Can you work these out from the model? Positions are in its coordinate system, mm. A direction names the side the tool comes from. Round coordinates to 2 decimals unless told otherwise and drop trailing zeros. Use a Markdown table: item, result.
from build123d import *

# Parameters (mm, degrees)
EXTRUDE1_DEPTH             = 250
EXTRUDE2_REACH             = 252.071
SKETCH2_R                  = 1.2
SKETCH_R                   = 2.1
SKETCH_R_2                 = 1.2
EXTRUDE4_DEPTH             = 2.3
CHAMFER1_SIZE              = 0.2
LPATTERN1_COUNT            = 17
LPATTERN1_PITCH            = 15
CHAMFER1_OF_LPATTERN1_SIZE = 0.2


with BuildPart() as part:
    # Sketch1 → Extrude1 (new body)
    with BuildSketch(Plane.XY):
        with BuildLine():
            Line((-3.3, -2.4), (3.3, -2.4))
            Line((3.3, -2.4), (3.5, -2.2))
            Line((3.5, -2.2), (3.5, 0.106274607))
            ThreePointArc((3.5, 0.106274607), (3.091294745, 0.282570681), (2.840065792, 0.65))
            Line((2.840065792, 0.65), (2.340065792, 0.65))
            Line((2.340065792, 0.65), (2.340065792, 1.15))
            Line((2.340065792, 1.15), (2.840065792, 1.15))
            ThreePointArc((2.840065792, 1.15), (3.091294745, 1.517429319), (3.5, 1.693725393))
            Line((3.5, 1.693725393), (3.5, 2.2))
            Line((3.5, 2.2), (3.3, 2.4))
            Line((3.3, 2.4), (-3.3, 2.4))
            Line((-3.3, 2.4), (-3.5, 2.2))
            Line((-3.5, 2.2), (-3.5, 1.693725393))
            ThreePointArc((-3.5, 1.693725393), (-3.091294745, 1.517429319), (-2.840065792, 1.15))
            Line((-2.840065792, 1.15), (-2.340065792, 1.15))
            Line((-2.340065792, 1.15), (-2.340065792, 0.65))
            Line((-2.340065792, 0.65), (-2.840065792, 0.65))
            ThreePointArc((-2.840065792, 0.65), (-3.091294745, 0.282570681), (-3.5, 0.106274607))
            Line((-3.5, 0.106274607), (-3.5, -2.2))
            Line((-3.5, -2.2), (-3.3, -2.4))
        make_face()
    extrude(amount=EXTRUDE1_DEPTH)

    # Sketch2 → Extrude2 (cut, up to next)
    with BuildSketch(Plane(origin=(0, 2.4, 0), x_dir=(1, 0, 0), z_dir=(0, 1, 0)), mode=Mode.PRIVATE) as extrude2_sk1:
        with Locations(Location((0, -5, 0), (0, 0, 270))):
            Circle(SKETCH2_R)
    extrude2_tool1 = extrude(extrude2_sk1.sketch, amount=-EXTRUDE2_REACH, mode=Mode.PRIVATE) & part.part
    extrude2 = extrude2_tool1.solids().sort_by_distance((0, 2.4, 5))[0]
    add(extrude2, mode=Mode.SUBTRACT)

    # Sketch → Extrude4 (cut)
    with BuildSketch(Plane(origin=(0, 2.4, 0), x_dir=(1, 0, 0), z_dir=(0, 1, 0))):
        with Locations(Location((0, -5, 0), (0, 0, 270))):
            Circle(SKETCH_R)
        with Locations(Location((0, -5, 0), (0, 0, 270))):
            Circle(SKETCH_R_2, mode=Mode.SUBTRACT)
    extrude4 = extrude(amount=-EXTRUDE4_DEPTH, mode=Mode.SUBTRACT)

    # Chamfer1
    chamfer1_edges = [part.edges().sort_by_distance(p)[0] for p in [
        (0, -2.4, 3.8),
        (0, 2.4, 2.9),
    ]]
    chamfer(chamfer1_edges, length=CHAMFER1_SIZE)

    # LPattern1: Extrude2, Extrude4 ×17
    with Locations(*[(0, 0, i * LPATTERN1_PITCH) for i in range(1, LPATTERN1_COUNT)]):
        add(extrude2, mode=Mode.SUBTRACT)
        add(extrude4, mode=Mode.SUBTRACT)

    # Chamfer1 of LPattern1
    chamfer1_of_lpattern1_edges = [part.edges().sort_by_distance(p)[0] for p in [
        (0, -2.4, 18.8),
        (0, 2.4, 17.9),
        (0, -2.4, 33.8),
        (0, 2.4, 32.9),
        (0, -2.4, 48.8),
        (0, 2.4, 47.9),
        (0, -2.4, 63.8),
        (0, 2.4, 62.9),
        (0, -2.4, 78.8),
        (0, 2.4, 77.9),
        (0, -2.4, 93.8),
        (0, 2.4, 92.9),
        (0, -2.4, 108.8),
        (0, 2.4, 107.9),
        (0, -2.4, 123.8),
        (0, 2.4, 122.9),
        (0, -2.4, 138.8),
        (0, 2.4, 137.9),
        (0, -2.4, 153.8),
        (0, 2.4, 152.9),
        (0, -2.4, 168.8),
        (0, 2.4, 167.9),
        (0, -2.4, 183.8),
        (0, 2.4, 182.9),
        (0, -2.4, 198.8),
        (0, 2.4, 197.9),
        (0, -2.4, 213.8),
        (0, 2.4, 212.9),
        (0, -2.4, 228.8),
        (0, 2.4, 227.9),
        (0, -2.4, 243.8),
        (0, 2.4, 242.9),
    ]]
    chamfer(chamfer1_of_lpattern1_edges, length=CHAMFER1_OF_LPATTERN1_SIZE)


solid = part.part
1. Which directions (+Z, -Z, +X, -X, +Y, -Y) give clear straight access to the entire face, cutting with the end or side of a thin tool? Please do faces 3 (the flat face through (0, -2.4, 123)), 4 (the cylindrical face through (0.631, 1.165, 127.003)).
Answer sheet:
| item | result |
|---|---|
| face 3 | +Z, -Z, +X, -X, -Y |
| face 4 | +Y |
2. I need wall thicknesses on line 1 (X direction, y = 1, z = 185); line 2 (X direction, y = -1.4, z = 80); line 3 (Y direction, x = 2, z = 36). Which ranges of each line are inside material? Lowest first, please.
Answer sheet:
| item | result |
|---|---|
| line 1 | x = -2.34 to -2.1, 2.1 to 2.34 |
| line 2 | x = -3.5 to -1.2, 1.2 to 3.5 |
| line 3 | y = -2.4 to 2.34 |
3. If we mould it in two halves opening along Z, with no side actions, what happens to faces 1 (the flat face through (2, 2.4, 123)), 2 (the cylindrical face through (0.09, 1.16, 92.9))? For each: +Z half, -Z half, draft (parallel to the pull), parting line (faces both ways), or undercut.
Answer sheet:
| item | result |
|---|---|
| face 1 | draft |
| face 2 | undercut |
4. Will these pins go through, and if not, where does the flat tip stop? pin 1 Ø2.5 at (x, z) = (0, 110) entering from -Y; pin 2 Ø1.3 at (x, z) = (1, 230) entering from +Y.
Answer sheet:
| item | result |
|---|---|
| pin 1 | stops at y = -2.25 |
| pin 2 | stops at y = 0.1 |
5. I want a section at A-A (x = 0). State how many separate pieces and enclosed holes the cut face has, plus the area to 3 significant figures.
Answer sheet:
| item | result |
|---|---|
| separate pieces | 18 |
| enclosed holes | 0 |
| area | 932 mm² |
